Design review of the part built by this model. Coordinates are the model's own, in mm. A direction names the side the tool comes from. Coordinates: 2 decimals unless noted, no trailing zeros. Write each loop counter-clockwise with the first axis right and the second up, starting at its lowest first coordinate (ties: lowest second). Pieces come first, ordered by that corner, then holes. Notation, with made-up numbers: (79, 66.5) - (106, 66.5) arc R30 ccw to (106, 88.5) - close; hole circle Ø7 at (40.5, 58.5). An arc over 180 degrees is marked (long way). One line per item, written item: value.
from build123d import *

# Parameters (mm, degrees)
F0_R        = 35
F1_DEPTH    = 7.5
F2_R        = 18.35
F3_DEPTH    = 25
F5_R        = 30
F5_R_2      = 20
F6_DEPTH    = 67.5
F7_R        = 5
F8_START    = 62.5
F6_FACE_R   = 20
F6_FACE_R_2 = 18.35
F8_DEPTH    = 5
F9_R        = 1
F11_R       = 18.35
F12_DEPTH   = 5
F13_R       = 35
F13_R_2     = 33.75
F14_DEPTH   = 2.5


with BuildPart() as f1:
    # F0 (on Top) → F1 (new body)
    with BuildSketch(Plane.XY):
        Circle(F0_R)
    extrude(amount=F1_DEPTH)

    # F2 (on face) → F3 (cut)
    with BuildSketch(Plane.XY.offset(7.5)):
        Circle(F2_R)
    extrude(amount=-F3_DEPTH, mode=Mode.SUBTRACT)

    # F5 (on face) → F6 (join)
    with BuildSketch(Plane.XY.offset(7.5)):
        Circle(F5_R)
        Circle(F5_R_2, mode=Mode.SUBTRACT)
    extrude(amount=F6_DEPTH)

    # F7
    f7_edges = [f1.edges().sort_by_distance(p)[0] for p in [
        (-30, 0, 75),
    ]]
    fillet(f7_edges, radius=F7_R)

    # F6_face (on face) → F8 (join)
    with BuildSketch(Plane.XY.offset(7.5).offset(F8_START)):
        Circle(F6_FACE_R)
        Circle(F6_FACE_R_2, mode=Mode.SUBTRACT)
    extrude(amount=F8_DEPTH)

    # F9
    f9_edges = [f1.edges().sort_by_distance(p)[0] for p in [
        (-35, 0, 7.5),
    ]]
    fillet(f9_edges, radius=F9_R)

    # F11 (on offset) → F12 (join)
    with BuildSketch(Plane.XY.offset(75)):
        Circle(F11_R)
    extrude(amount=-F12_DEPTH)

    # F13 (on face) → F14 (join)
    with BuildSketch(Plane.XY):
        Circle(F13_R)
        Circle(F13_R_2, mode=Mode.SUBTRACT)
    extrude(amount=-F14_DEPTH)


solid = f1.part
1. Wall thickness on line 1 along Y through (x, z) = (0, 44.5); line 2 along Y through (x, z) = (0, -1.6); line 3 along Z through (x, y) = (29, -8): over which ranges is each line inside the solid? List them lowest first.
Answer block:
line 1: y = -30 to -20, 20 to 30
line 2: y = -35 to -33.75, 33.75 to 35
line 3: z = 0 to 7.5
2. For faces 1 (the face through (-18, 29, -2.5)), 2 (the face through (-28, -21, 2)), 3 (the face through (2.4, -30.1, 7.5)), 4 (the face through (15, -15, 0)), 5 (the face through (18, -6, 7.5)), list the 3-axis set-ups (+Z, -Z, +X, -X, +Y, -Y) from which the entire face can be reached by the end or side of a thin tool; tool diameter is ignored.
Answer block:
face 1: -Z, +X, -X, +Y, -Y
face 2: +Z, -Z
face 3: +Z
face 4: -Z
face 5: none
3. Consider section A-A, the plane y = 0. Write out the cut boundary in (x, z), then the cut area to 3 significant figures.
Answer block:
outline: (-35, -2.5) - (-33.75, -2.5) - (-33.75, 0) - (-18.35, 0) - (-18.35, 7.5) - (-20, 7.5) - (-20, 70) - (20, 70) - (20, 7.5) - (18.35, 7.5) - (18.35, 0) - (33.75, 0) - (33.75, -2.5) - (35, -2.5) - (35, 6.5) arc R1 ccw to (34, 7.5) - (30, 7.5) - (30, 70) arc R5 ccw to (25, 75) - (-25, 75) arc R5 ccw to (-30, 70) - (-30, 7.5) - (-34, 7.5) arc R1 ccw to (-35, 6.5) - close
area: 1,790 mm^2
4. Consider section C-C, the plane z = 9. Write out the cut boundary in (x, y).
Answer block:
outline: circle Ø60 at (0, 0); hole circle Ø40 at (0, 0)
5. Mouldability with a two-part tool opening along X and no side actions: class faces 6 (the face through (-4.336, -19.524, 38.312)), 7 (the face through (-29.97, 1.32, 38.31)), 8 (the face through (0, 0, 75)) as released by +X, released by -X, zero draft, split by the parting line, or undercut.
Answer block:
face 6: undercut
face 7: split by the parting line
face 8: zero draft
6. Insertion check: pin 1 Ø5 at (y, z) = (7.5, 31) entering from -X; pin 2 Ø2 at (x, z) = (-5.5, 44) entering from +Y; pin 3 Ø1 at (x, z) = (26.5, 37.5) entering from +Y. Each pin has a flat end and moves straight along its axis. Give the tip position at first contact, or say it passes through.
Answer block:
pin 1: stops at x = -29.58
pin 2: stops at y = 29.66
pin 3: stops at y = 14.97
